Work out the finished part from the listing and answer in its coordinate system (mm). Give positions to 0.01 mm unless a question says otherwise; leave off trailing zeros. Loops run counter-clockwise (first coordinate to the right, second up) from the corner with the lowest first, then second, coordinate; pieces in that order, holes last. Notation, with made-up numbers: (12, 54) -> (59, 54) arc R20 ccw to (59, 73) -> close; hole circle Ø9 at (-29, 8.25). An arc over 180 degrees is marked (long way). Answer as CSV lines item,"result". Start each with the question number.
1. Find section C-C, the plane y = 61.5. Give the vertices of the cut face in (x, z), and give its area (3 significant figures).
2. A flat-ended cylindrical pin translates along its axis: pin 1 Ø1.5 at (x, z) = (-121, 15) entering from +Y. Find the tip coordinate at first contact, or state that the pin passes through.
3. Determine the mould class of faces 1 (the face through (-121.849, 19.976, -8.955)), 2 (the face through (-122, 0, 0)), 3 (the face through (-122, 34, 33.35)) for opening direction Y: +Y half, -Y half, draft (parallel to the pull), parting line (faces both ways), or undercut.
4. Find section B-B, the plane x = -122.5. Give the vertices of the cut face in (y, z) (3 decimals).
5. Find section A-A, the plane y = 6. Give the vertices of the cut face in (x, z), and give its area (3 significant figures).
6. Find the intervals of material crossed by line 1 along Z through (x, y) = (-121.35, 21) (3 decimals); line 2 along Y through (x, z) = (-123.5, 7.5), in increasing order.
from build123d import *

# Parameters (mm, degrees)
SKETCH_1_W                   = 40
SKETCH_1_H                   = 66.7
EXTRUDE_1_DEPTH              = 2
SKETCH_2_W                   = 4
SKETCH_2_H                   = 66.7
EXTRUDE_2_DEPTH              = 100
CUT_EXTRUDE_1_DEPTH          = 115.526077816
CUT_EXTRUDE_1_DEPTH_BACK     = 115.526077816
HOLE_WIZARD_M4_1_D           = 3.3
HOLE_WIZARD_M4_1_CSINK_D     = 4.05
HOLE_WIZARD_M4_1_CSINK_ANGLE = 90
HOLE_WIZARD_M4_2_AT_2_COUNT  = 2
HOLE_WIZARD_M4_2_AT_2_PITCH  = 68.59294731
HOLE_WIZARD_M4_2_AT_3_COUNT  = 2
HOLE_WIZARD_M4_2_AT_3_PITCH  = 26
HOLE_WIZARD_M4_2_AT_4_COUNT  = 2
HOLE_WIZARD_M4_2_AT_4_PITCH  = 62.376998966
HOLE_WIZARD_M4_2_AT_5_COUNT  = 2
HOLE_WIZARD_M4_2_AT_5_PITCH  = 56.7
SKETCH_11_W                  = 66.7
SKETCH_11_H                  = 2
EXTRUDE_3_DEPTH              = 100
SKETCH_13_W                  = 40
SKETCH_13_H                  = 66.7
EXTRUDE_4_DEPTH              = 2
SKETCH_14_W                  = 4
SKETCH_14_H                  = 66.7
EXTRUDE_5_DEPTH              = 100
CUT_EXTRUDE_2_DEPTH          = 180.589037806
CUT_EXTRUDE_2_DEPTH_BACK     = 180.589037806
HOLE_WIZARD_M4_3_AT_2_COUNT  = 2
HOLE_WIZARD_M4_3_AT_2_PITCH  = 26
HOLE_WIZARD_M4_3_AT_3_COUNT  = 2
HOLE_WIZARD_M4_3_AT_3_PITCH  = 62.376998966
HOLE_WIZARD_M4_3_AT_4_COUNT  = 2
HOLE_WIZARD_M4_3_AT_4_PITCH  = 56.7
CUT_EXTRUDE_3_REACH          = 181.589
SKETCH_18_R                  = 9.5
CUT_EXTRUDE_4_REACH          = 181.589
SKETCH_21_R                  = 11
CUT_EXTRUDE_5_REACH          = 181.589
SKETCH_22_R                  = 4.5
FILLET_1_R                   = 2
CUT_EXTRUDE_6_REACH          = 193.604
SKETCH_23_W                  = 36
SKETCH_23_H                  = 66.7
CUT_EXTRUDE_7_REACH          = 164.752
SKETCH_24_W                  = 36
SKETCH_24_H                  = 66.7
HOLE_WIZARD_M3_1_D           = 2.5
HOLE_WIZARD_M3_1_CSINK_D     = 3.05
HOLE_WIZARD_M3_1_CSINK_ANGLE = 90
CUT_EXTRUDE_8_DEPTH          = 154.990981879
CUT_EXTRUDE_8_DEPTH_BACK     = 154.990981879
SKETCH_27_W                  = 104
SKETCH_27_H                  = 66.7
FILLET_2_R                   = 0.8


# Read off the part's stored shape, not the designer's step: the hole wizard step, the hole wizard step
with BuildPart() as part:
    # Sketch 1 → Extrude 1 (new body)
    with BuildSketch(Plane(origin=(0, 0, 0), x_dir=(1, 0, 0), z_dir=(0, 1, 0))):
        Rectangle(SKETCH_1_W, SKETCH_1_H)
    extrude(amount=EXTRUDE_1_DEPTH)

    # Sketch 2 → Extrude 2 (add)
    with BuildSketch(Plane(origin=(0, 2, 0), x_dir=(1, 0, 0), z_dir=(0, 1, 0))):
        with Locations((-18, 0)):
            Rectangle(SKETCH_2_W, SKETCH_2_H)
    extrude(amount=EXTRUDE_2_DEPTH)

    # Sketch 5 → Cut-Extrude 1 (cut, two sides: drawn at the far end of the back side and taken through both)
    with BuildSketch(Plane.ZY.offset(20).offset(-CUT_EXTRUDE_1_DEPTH_BACK)):
        with BuildLine():
            ThreePointArc((0, 102), (23.582011153, 92.232011153), (33.35, 68.65))
            Line((33.35, 68.65), (33.35, 102))
            Line((33.35, 102), (0, 102))
        make_face()
        with BuildLine():
            ThreePointArc((-33.35, 68.65), (-23.582011153, 92.232011153), (0, 102))
            Line((0, 102), (-33.35, 102))
            Line((-33.35, 102), (-33.35, 68.65))
        make_face()
    extrude(amount=CUT_EXTRUDE_1_DEPTH + CUT_EXTRUDE_1_DEPTH_BACK, mode=Mode.SUBTRACT)

    # Hole Wizard M4 _1 (through all)
    with Locations(Plane.ZY.offset(20)):
        with Locations((0, 97.65), (25.11473671, 54.15), (-25.11473671, 54.15)):
            CounterSinkHole(HOLE_WIZARD_M4_1_D / 2, HOLE_WIZARD_M4_1_CSINK_D / 2, counter_sink_angle=HOLE_WIZARD_M4_1_CSINK_ANGLE)

    # Sketch 10 → Hole Wizard M4 _2 (revolve, cut)
    with BuildSketch(Plane(origin=(15, 2, -28.35), x_dir=(0, 0, 1), z_dir=(1, 0, 0))):
        Polygon((0, 0), (0, 2), (1.65, 2), (1.65, 0.375), (2.025, 0), align=None)
    hole_wizard_m4_2 = revolve(axis=Axis((15, 8.35, -28.35), (0, -1, 0)), mode=Mode.SUBTRACT)

    # Hole Wizard M4 _2 at 2: Hole Wizard M4 _2 ×2
    with Locations(*[Vector(-0.9508085645250022, 0, 0.3097790722852413) * (i * HOLE_WIZARD_M4_2_AT_2_PITCH) for i in range(1, HOLE_WIZARD_M4_2_AT_2_COUNT)]):
        add(hole_wizard_m4_2, mode=Mode.SUBTRACT)

    # Hole Wizard M4 _2 at 3: Hole Wizard M4 _2 ×2
    with Locations(*[(-i * HOLE_WIZARD_M4_2_AT_3_PITCH, 0, 0) for i in range(1, HOLE_WIZARD_M4_2_AT_3_COUNT)]):
        add(hole_wizard_m4_2, mode=Mode.SUBTRACT)

    # Hole Wizard M4 _2 at 4: Hole Wizard M4 _2 ×2
    with Locations(*[Vector(-0.4168203092647413, 0, 0.9089889052042635) * (i * HOLE_WIZARD_M4_2_AT_4_PITCH) for i in range(1, HOLE_WIZARD_M4_2_AT_4_COUNT)]):
        add(hole_wizard_m4_2, mode=Mode.SUBTRACT)

    # Hole Wizard M4 _2 at 5: Hole Wizard M4 _2 ×2
    with Locations(*[(0, 0, i * HOLE_WIZARD_M4_2_AT_5_PITCH) for i in range(1, HOLE_WIZARD_M4_2_AT_5_COUNT)]):
        add(hole_wizard_m4_2, mode=Mode.SUBTRACT)

    # Sketch 11 → Extrude 3 (add)
    with BuildSketch(Plane.ZY.offset(20)):
        with Locations((0, 16)):
            Rectangle(SKETCH_11_W, SKETCH_11_H)
    extrude(amount=EXTRUDE_3_DEPTH)



with BuildPart() as body_2:
    # Sketch 13 → Extrude 4 (new body)
    with BuildSketch(Plane(origin=(0, 0, 0), x_dir=(1, 0, 0), z_dir=(0, 1, 0))):
        with Locations((-140, 0)):
            Rectangle(SKETCH_13_W, SKETCH_13_H)
    extrude(amount=EXTRUDE_4_DEPTH)


with BuildPart() as part_1:
    add(part.part)

    add(body_2.part)  # Extrude 5 merges body 2
    # Sketch 14 → Extrude 5 (add)
    with BuildSketch(Plane(origin=(0, 2, 0), x_dir=(1, 0, 0), z_dir=(0, 1, 0))):
        with Locations((-122, 0)):
            Rectangle(SKETCH_14_W, SKETCH_14_H)
    extrude(amount=EXTRUDE_5_DEPTH)

    # Sketch 15 → Cut-Extrude 2 (cut, two sides: drawn at the far end of the back side and taken through both)
    with BuildSketch(Plane.ZY.offset(124).offset(-CUT_EXTRUDE_2_DEPTH_BACK)):
        with BuildLine():
            ThreePointArc((0, 102), (23.582011153, 92.232011153), (33.35, 68.65))
            Line((33.35, 68.65), (33.35, 102))
            Line((33.35, 102), (0, 102))
        make_face()
        with BuildLine():
            ThreePointArc((-33.35, 68.65), (-23.582011153, 92.232011153), (0, 102))
            Line((0, 102), (-33.35, 102))
            Line((-33.35, 102), (-33.35, 68.65))
        make_face()
    extrude(amount=CUT_EXTRUDE_2_DEPTH + CUT_EXTRUDE_2_DEPTH_BACK, mode=Mode.SUBTRACT)

    # Sketch 17 → Hole Wizard M4 _3 (revolve, cut)
    with BuildSketch(Plane(origin=(-129, 2, -28.35), x_dir=(0, 0, 1), z_dir=(1, 0, 0))):
        Polygon((0, 0), (0, 2), (1.65, 2), (1.65, 0.375), (2.025, 0), align=None)
    hole_wizard_m4_3 = revolve(axis=Axis((-129, 8.35, -28.35), (0, -1, 0)), mode=Mode.SUBTRACT)

    # Hole Wizard M4 _3 at 2: Hole Wizard M4 _3 ×2
    with Locations(*[(-i * HOLE_WIZARD_M4_3_AT_2_PITCH, 0, 0) for i in range(1, HOLE_WIZARD_M4_3_AT_2_COUNT)]):
        add(hole_wizard_m4_3, mode=Mode.SUBTRACT)

    # Hole Wizard M4 _3 at 3: Hole Wizard M4 _3 ×2
    with Locations(*[Vector(-0.41682030926474106, 0, 0.9089889052042636) * (i * HOLE_WIZARD_M4_3_AT_3_PITCH) for i in range(1, HOLE_WIZARD_M4_3_AT_3_COUNT)]):
        add(hole_wizard_m4_3, mode=Mode.SUBTRACT)

    # Hole Wizard M4 _3 at 4: Hole Wizard M4 _3 ×2
    with Locations(*[(0, 0, i * HOLE_WIZARD_M4_3_AT_4_PITCH) for i in range(1, HOLE_WIZARD_M4_3_AT_4_COUNT)]):
        add(hole_wizard_m4_3, mode=Mode.SUBTRACT)

    # Sketch 18 → Cut-Extrude 3 (cut, up to next)
    with BuildSketch(Plane.ZY.offset(124), mode=Mode.PRIVATE) as cut_extrude_3_sk1:
        with Locations((0, 68.65)):
            Circle(SKETCH_18_R)
    cut_extrude_3_tool1 = extrude(cut_extrude_3_sk1.sketch, amount=-CUT_EXTRUDE_3_REACH, mode=Mode.PRIVATE) & part_1.part
    add(cut_extrude_3_tool1.solids().sort_by_distance((-124, 68.65, 0))[0], mode=Mode.SUBTRACT)

    # Sketch 21 → Cut-Extrude 4 (cut, up to next)
    with BuildSketch(Plane(origin=(-16, 0, 0), x_dir=(0, 0, -1), z_dir=(1, 0, 0)), mode=Mode.PRIVATE) as cut_extrude_4_sk1:
        with Locations((0, 68.65)):
            Circle(SKETCH_21_R)
    cut_extrude_4_tool1 = extrude(cut_extrude_4_sk1.sketch, amount=-CUT_EXTRUDE_4_REACH, mode=Mode.PRIVATE) & part_1.part
    add(cut_extrude_4_tool1.solids().sort_by_distance((-16, 68.65, 0))[0], mode=Mode.SUBTRACT)

    # Sketch 22 → Cut-Extrude 5 (cut, up to next)
    with BuildSketch(Plane(origin=(-16, 0, 0), x_dir=(0, 0, -1), z_dir=(1, 0, 0)), mode=Mode.PRIVATE) as cut_extrude_5_sk1:
        with Locations((16.670989023, 59.025)):
            Circle(SKETCH_22_R)
    cut_extrude_5_tool1 = extrude(cut_extrude_5_sk1.sketch, amount=-CUT_EXTRUDE_5_REACH, mode=Mode.PRIVATE) & part_1.part
    add(cut_extrude_5_tool1.solids().sort_by_distance((-16, 59.025, -16.670989))[0], mode=Mode.SUBTRACT)

    # Fillet 1
    fillet_1_edges = [part_1.edges().sort_by_distance(p)[0] for p in [
        (-160, 1, -33.35),
        (-160, 1, 33.35),
        (20, 1, 33.35),
        (20, 1, -33.35),
    ]]
    fillet(fillet_1_edges, radius=FILLET_1_R)

    # Sketch 23 → Cut-Extrude 6 (cut, up to next)
    with BuildSketch(Plane(origin=(0, 2, 0), x_dir=(1, 0, 0), z_dir=(0, 1, 0)), mode=Mode.PRIVATE) as cut_extrude_6_sk1:
        with Locations((-142, 0)):
            Rectangle(SKETCH_23_W, SKETCH_23_H)
    cut_extrude_6_tool1 = extrude(cut_extrude_6_sk1.sketch, amount=-CUT_EXTRUDE_6_REACH, mode=Mode.PRIVATE) & part_1.part
    add(cut_extrude_6_tool1.solids().sort_by_distance((-142, 2, 0))[0], mode=Mode.SUBTRACT)

    # Sketch 24 → Cut-Extrude 7 (cut, up to next)
    with BuildSketch(Plane(origin=(0, 2, 0), x_dir=(1, 0, 0), z_dir=(0, 1, 0)), mode=Mode.PRIVATE) as cut_extrude_7_sk1:
        with Locations((2, 0)):
            Rectangle(SKETCH_24_W, SKETCH_24_H)
    cut_extrude_7_tool1 = extrude(cut_extrude_7_sk1.sketch, amount=-CUT_EXTRUDE_7_REACH, mode=Mode.PRIVATE) & part_1.part
    add(cut_extrude_7_tool1.solids().sort_by_distance((2, 2, 0))[0], mode=Mode.SUBTRACT)

    # Hole Wizard M3 _1 (through all)
    with Locations(Plane(origin=(-16, 0, 0), x_dir=(0, 0, -1), z_dir=(1, 0, 0))):
        with Locations((9, 6), (-9, 6)):
            CounterSinkHole(HOLE_WIZARD_M3_1_D / 2, HOLE_WIZARD_M3_1_CSINK_D / 2, counter_sink_angle=HOLE_WIZARD_M3_1_CSINK_ANGLE)

    # Sketch 27 → Cut-Extrude 8 (cut, two sides: drawn at the far end of the back side and taken through both)
    with BuildSketch(Plane(origin=(0, 17, 0), x_dir=(1, 0, 0), z_dir=(0, 1, 0)).offset(-CUT_EXTRUDE_8_DEPTH_BACK)):
        with Locations((-68, 0)):
            Rectangle(SKETCH_27_W, SKETCH_27_H)
    extrude(amount=CUT_EXTRUDE_8_DEPTH + CUT_EXTRUDE_8_DEPTH_BACK, mode=Mode.SUBTRACT)

    # Hole Wizard M2.5 _1 outline → Hole Wizard M2.5 _1 (revolve, cut)
    with BuildSketch(Plane(origin=(0, 21, -9), x_dir=(0, 1, 0), z_dir=(0, 0, -1))):
        Polygon((1.025, -123.75), (1.025, -120), (0, -120), (0, -124), (1.275, -124), align=None)
    revolve(axis=Axis((0, 21, -9), (1, 0, 0)), mode=Mode.SUBTRACT)

    # Hole Wizard M2.5 _1 2 outline → Hole Wizard M2.5 _1 2 (revolve, cut)
    with BuildSketch(Plane(origin=(0, 21, 9), x_dir=(0, 1, 0), z_dir=(0, 0, -1))):
        Polygon((1.025, -123.75), (1.025, -120), (0, -120), (0, -124), (1.275, -124), align=None)
    revolve(axis=Axis((0, 21, 9), (1, 0, 0)), mode=Mode.SUBTRACT)

    # Fillet 2
    fillet_2_edges = [part_1.edges().sort_by_distance(p)[0] for p in [
        (-120, 34.325, 33.35),
        (-120, 34.325, -33.35),
        (-122, 0, -33.35),
        (-124, 34.325, -33.35),
        (-120, 102, 0),
        (-124, 102, 0),
        (-124, 34.325, 33.35),
    ]]
    fillet(fillet_2_edges, radius=FILLET_2_R)

    # Hole Wizard M1.6 _1 outline → Hole Wizard M1.6 _1 (revolve, cut)
    with BuildSketch(Plane(origin=(0, 75, 28.85), x_dir=(0, 1, 0), z_dir=(0, 0, -1))):
        Polygon((0.625, -123.8), (0.625, -120), (0, -120), (0, -124), (0.825, -124), align=None)
    revolve(axis=Axis((0, 75, 28.85), (1, 0, 0)), mode=Mode.SUBTRACT)

    # Hole Wizard M1.6 _1 2 outline → Hole Wizard M1.6 _1 2 (revolve, cut)
    with BuildSketch(Plane(origin=(0, 78.6, 28.85), x_dir=(0, 1, 0), z_dir=(0, 0, -1))):
        Polygon((0.625, -123.8), (0.625, -120), (0, -120), (0, -124), (0.825, -124), align=None)
    revolve(axis=Axis((0, 78.6, 28.85), (1, 0, 0)), mode=Mode.SUBTRACT)


solid = part_1.part
Resolved:
1,outline,"(-124, -32.55) arc R0.8 ccw to (-123.2, -33.35) -> (-120.8, -33.35) arc R0.8 ccw to (-120, -32.55) -> (-120, -6.26) -> (-124, -6.26) -> close; (-124, 6.26) -> (-120, 6.26) -> (-120, 32.55) arc R0.8 ccw to (-120.8, 33.35) -> (-123.2, 33.35) arc R0.8 ccw to (-124, 32.55) -> close"
1,area,"216 mm^2"
2,pin 1,"stops at y = 98.8"
3,face 1,"undercut"
3,face 2,"-Y half"
3,face 3,"draft"
4,outline,"(0, -32.55) arc R0.8 ccw to (0.8, -33.35) -> (68.65, -33.35) arc R33.35 ccw to (68.65, 33.35) -> (0, 33.35) -> close; hole circle Ø2.5 at (6, -9); hole circle Ø2.5 at (6, 9); hole circle Ø2.05 at (21, -9); hole circle Ø2.05 at (21, 9); hole circle Ø19 at (68.65, 0); hole circle Ø1.25 at (75, 28.85); hole circle Ø1.25 at (78.6, 28.85)"
5,outline,"(-124, -32.55) arc R0.8 ccw to (-123.2, -33.35) -> (-120.8, -33.35) arc R0.8 ccw to (-120, -32.55) -> (-120, -10.25) -> (-124, -10.25) -> close; (-124, -7.75) -> (-120, -7.75) -> (-120, 7.75) -> (-124, 7.75) -> close; (-124, 10.25) -> (-120, 10.25) -> (-120, 32.55) arc R0.8 ccw to (-120.8, 33.35) -> (-123.2, 33.35) arc R0.8 ccw to (-124, 32.55) -> close"
5,area,"246 mm^2"
6,line 1,"z = -33.35 to -10.025, -7.975 to 7.975, 10.025 to 33.35"
6,line 2,"y = 0 to 62.82, 74.48 to 101.09"
